Could you check a few things on this drawing? It's one solid part, dimensions in mm from its lowest x, y, z. A direction names the side the tool comes from. Coordinates: 2 decimals unless noted, no trailing zeros. Write each loop counter-clockwise with the first axis right and the second up, starting at its lowest first coordinate (ties: lowest second). Pieces come first, ordered by that corner, then holes. Notation, with made-up numbers: (53, -5) - (68, -5) arc R11 ccw to (68, 1) - close; hole circle Ø7 at (88.25, -3). An arc over 180 degrees is marked (long way). Answer as a JSON object with one key per item and string values. Group by question number.
1) If we section it at A-A (x = 23): Write out the boundary of the cut face in (y, z), plus the area to 3 significant figures.
2) If we section it at C-C (z = 15): Write out the boundary of the cut face in (x, y).
3) Will these pins go through, and if not, where does the flat tip stop? pin 1 Ø12 at (x, z) = (39.5, 40.5) entering from +Y; pin 2 Ø1 at (x, y) = (6.5, 14) entering from +Z; pin 3 Ø12 at (y, z) = (14.5, 16.5) entering from +X; pin 4 Ø6 at (x, y) = (18.5, 28) entering from +Z.
4) If we section it at B-B (y = 28.5): Write out the boundary of the cut face in (x, z), plus the area to 3 significant figures.
5) If we section it at D-D (x = 44): Write out the boundary of the cut face in (y, z), plus the area to 3 significant figures.
6) We'd pull the mould along Y, two halves only. Please class the marked faces 1, 2, 3 and 4: released by +Y, released by -Y, zero draft, split by the parting line, or undercut.
7) On a 3-axis mill with a long thin cutter (end or side, diameter ignored), from which of +Z, -Z, +X, -X, +Y, -Y can I reach the whole of each face in a straight line? I mean the marked faces 5 and 6. Say none if no direction works.
8) Please list where these lines run through material, in increasing order: line 1 along Y through (x, z) = (29, 13); line 2 along Z through (x, y) = (34, 25).
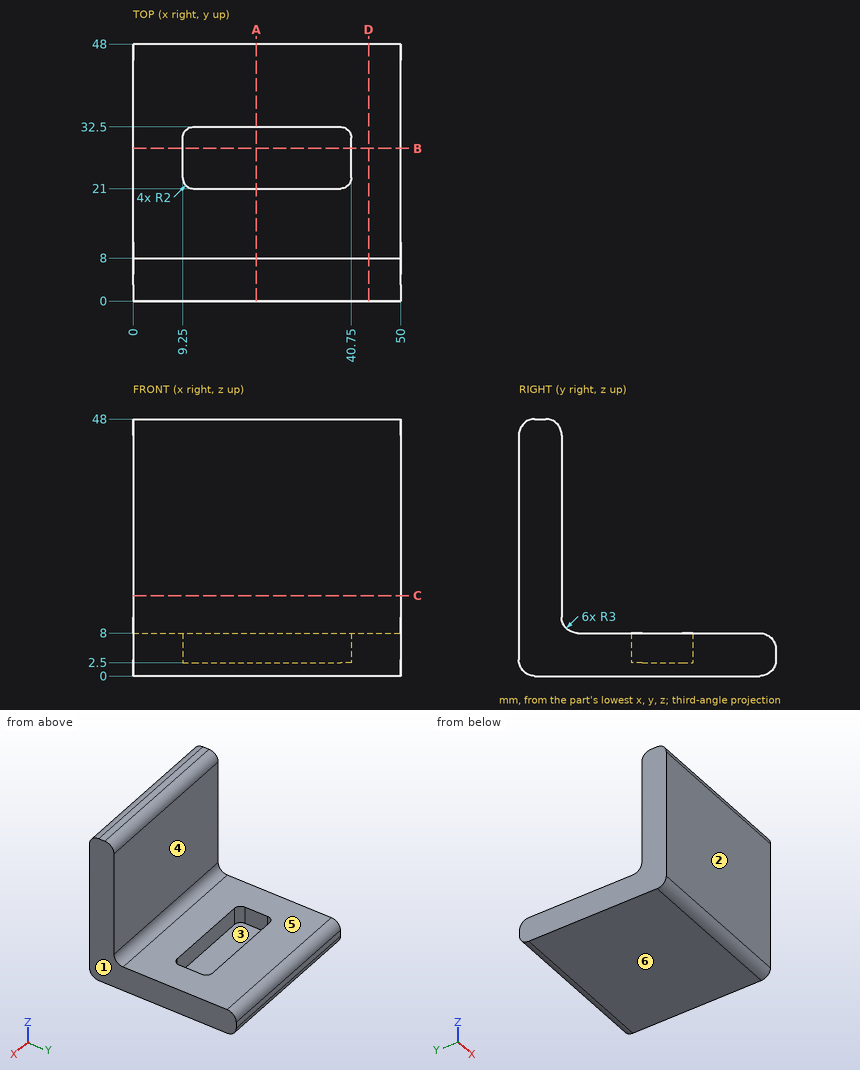
Here are the results:
{
 "1": {"outline": "(0, 3) arc R3 ccw to (3, 0) - (45, 0) arc R3 ccw to (48, 3) - (48, 5) arc R3 ccw to (45, 8) - (32.5, 8) - (32.5, 2.5) - (21, 2.5) - (21, 8) - (11, 8) arc R3 cw to (8, 11) - (8, 45) arc R3 ccw to (5, 48) - (3, 48) arc R3 ccw to (0, 45) - close", "area": "633 mm²"},
 "2": {"outline": "(0, 0) - (50, 0) - (50, 8) - (0, 8) - close"},
 "3": {"pin 1": "stops at y = 8", "pin 2": "stops at z = 8", "pin 3": "passes through", "pin 4": "stops at z = 2.5"},
 "4": {"outline": "(0, 0) - (50, 0) - (50, 8) - (40.75, 8) - (40.75, 2.5) - (9.25, 2.5) - (9.25, 8) - (0, 8) - close", "area": "227 mm²"},
 "5": {"outline": "(0, 3) arc R3 ccw to (3, 0) - (45, 0) arc R3 ccw to (48, 3) - (48, 5) arc R3 ccw to (45, 8) - (11, 8) arc R3 cw to (8, 11) - (8, 45) arc R3 ccw to (5, 48) - (3, 48) arc R3 ccw to (0, 45) - close", "area": "696 mm²"},
 "6": {"face 1": "zero draft", "face 2": "released by -Y", "face 3": "undercut", "face 4": "released by +Y"},
 "7": {"face 5": "+Z, +X, -X, +Y", "face 6": "-Z, +X, -X, +Y, -Y"},
 "8": {"line 1": "y = 0 to 8", "line 2": "z = 0 to 2.5"}
}
